Drawing for the job (mm, zero at the part's lowest x, y, z). Round coordinates to 2 decimals unless told otherwise and drop trailing zeros. Put each result on its own line as item: value. Start each with the question number.
Item 1: Probe probe 1 along Y at (x, z) = (20, 2.05) (1 decimal); probe 2 along Y at (x, z) = (69, 2.4) (1 decimal); probe 3 along X at (y, z) = (5, 1.8) (1 decimal). List the from-to ranges inside material, lowest first.
Item 2: Saw through at A-A on z = 2.6. State how many separate pieces and enclosed holes the cut face has, plus the area to 3 significant figures.
Item 3: Pin check, flat tips, straight feed: pin 1 Ø3.5 at (x, y) = (70.04, 17.21) entering from +Z (1 decimal); pin 2 Ø3.5 at (x, y) = (52.13, 63.69) entering from -Z. Stop position of each tip, or through.
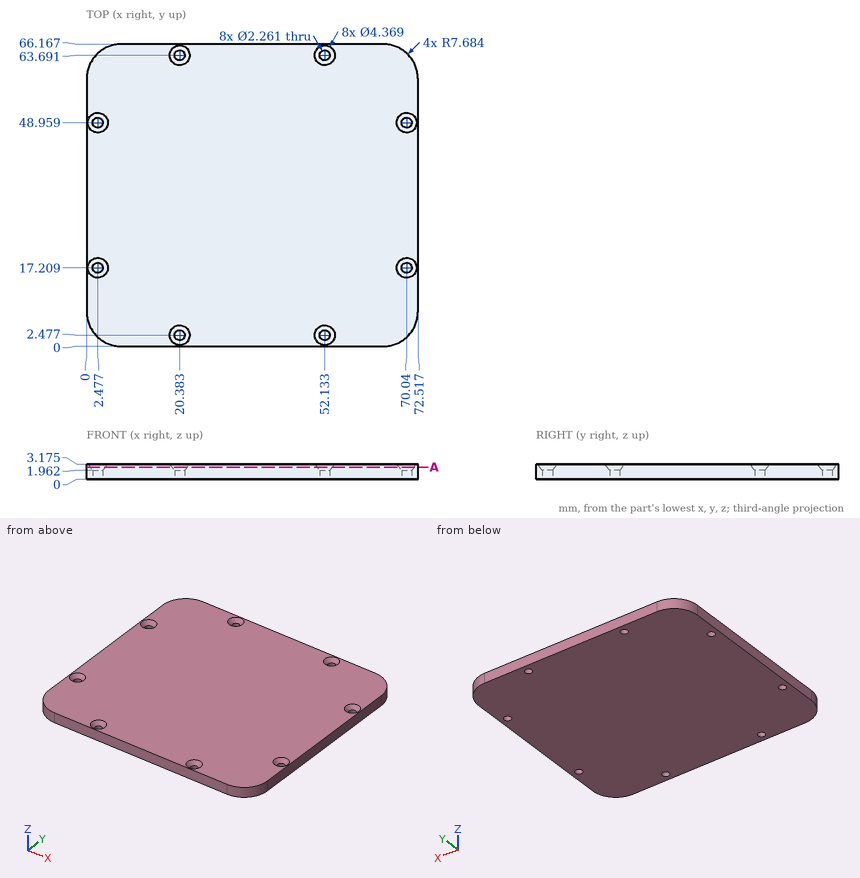
Results found:
1. probe 1: y = 0 to 1.3, 3.6 to 62.5, 64.8 to 66.2
1. probe 2: y = 1.2 to 16.1, 18.3 to 47.9, 50.1 to 64.9
1. probe 3: x = 0.5 to 72
2. separate pieces: 1
2. enclosed holes: 8
2. area: 4,680 mm²
3. pin 1: stops at z = 2.7
3. pin 2: stops at z = 0
